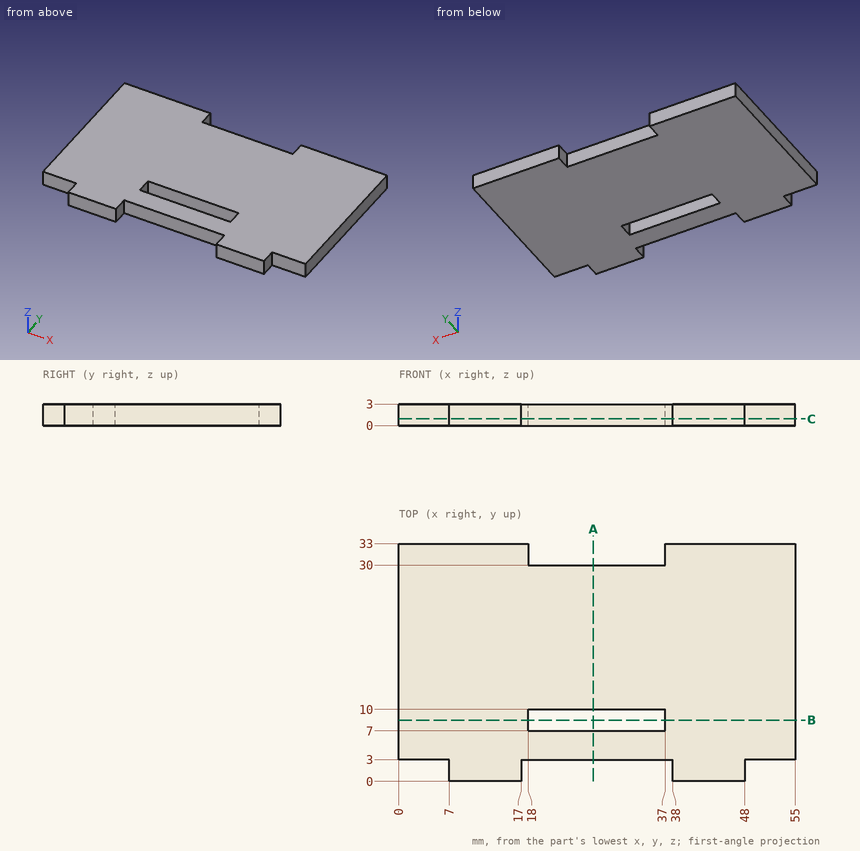
Print and shaded views of the part. All mm, measured from the part's lowest x, y and z. Give positions to 0.01 mm unless a question says otherwise; leave off trailing zeros. Order: outer loops, then holes, each group sorted by start corner. A loop starts at its lowest first (then second) coordinate and runs counter-clockwise, first axis right, second up. Notation, with made-up numbers: (34.25, 58.5) - (45.25, 58.5) arc R25 ccw to (45.25, 80.5) - close; hole circle Ø4 at (60, 53.5). An arc over 180 degrees is marked (long way). Use a Markdown table: item, result.
1) Saw through at B-B on y = 8.5. List the corners of the cut face in (x, z).
Checked values:
| item | result |
|---|---|
| outline | (0, 0) - (18, 0) - (18, 3) - (0, 3) - close; (37, 0) - (55, 0) - (55, 3) - (37, 3) - close |
2) Saw through at A-A on x = 27. List the corners of the cut face in (y, z).
Checked values:
| item | result |
|---|---|
| outline | (3, 0) - (7, 0) - (7, 3) - (3, 3) - close; (10, 0) - (30, 0) - (30, 3) - (10, 3) - close |
3) Flat gauge pins, fed straight in: P1, Ø12, axis at x = 25, y = 17, coming from the -Z side; P2, Ø0.9, axis at y = 2, z = 1, coming from the +X side; P3, Ø1.5, axis at x = 28, z = 2, coming from the -Y side; P4, Ø0.9, axis at x = 31, z = 2, coming from the +Y side. Where does each tip first touch, or does it go through?
Checked values:
| item | result |
|---|---|
| P1 | z = 0 |
| P2 | x = 48 |
| P3 | y = 3 |
| P4 | y = 30 |
4) Probe L1, parallel to Y at x = 21, z = 2.9; L2, parallel to Y at x = 4, z = 1.1. List the from-to ranges inside material, lowest first. Write a range as from..to.
Checked values:
| item | result |
|---|---|
| L1 | 3..7, 10..30 |
| L2 | 3..33 |
5) Saw through at C-C on z = 0.95. List the corners of the cut face in (x, y), plus the area to 3 significant figures.
Checked values:
| item | result |
|---|---|
| outline | (0, 3) - (7, 3) - (7, 0) - (17, 0) - (17, 3) - (38, 3) - (38, 0) - (48, 0) - (48, 3) - (55, 3) - (55, 33) - (37, 33) - (37, 30) - (18, 30) - (18, 33) - (0, 33) - close; hole (18, 7) - (37, 7) - (37, 10) - (18, 10) - close |
| area | 1,600 mm² |
